Autodesk Fusion 360 part; units mm, degrees
sketch "Sketch5" plane through (0, 0, 0) normal (0, 0, 1) x (1, 0, 0)
  line L0 (9.3481, 1.8494) -> (4.1024, 1.8494)
  line L1 (9.3481, -1.8494) -> (4.1024, -1.8494)
  arc A0 (9.2519, -1.8494) -> (9.2519, 1.8494) centre (9.3, 0) ccw
  arc A1 (4.1024, 1.8494) -> (4.1024, -1.8494) centre (0, 0) ccw
  dimension "d23" = 9
  dimension "d24" = 3.7
  dimension "d25" = 9.3
sketch "Sketch6" plane through (0, 0, 0) normal (0, 0, 1) x (1, 0, 0)
  circle A0 centre (0, 0) radius 1.7
  dimension "d26" = 3.4
extrude "Extrude6" add sketch "Sketch5" against normal blind 2.7
hole "Hole2" at (0, 0, 0) direction (0, 0, -1) diameter 3.4 depth 2.7 tip angle 118
sketch "Sketch7" plane through (0, 0, 0) normal (0, 0, 1) x (1, 0, 0)
  circle A0 centre (9.3, 0) radius 1.55
  dimension "d32" = 3.1
  dimension "d33" = 9.3
extrude "Extrude7" add sketch "Sketch7" along normal blind 10.4
sketch "Sketch1" plane through (0, 0, 0) normal (0, 0, 1) x (1, 0, 0)
  circle A0 centre (0, 0) radius 10.7065
  dimension "d1" = 21.413
extrude "Extrude1" [suppressed]
sketch "Sketch2" plane through (0, 0, 0) normal (0, 0, 1) x (1, 0, 0)
  circle A0 centre (0, 0) radius 1.5
  dimension "d4" = 3
sketch "Sketch3" plane through (0, 0, 0) normal (0, 0, 1) x (1, 0, 0)
  circle A0 centre (0, 0) radius 1.5
  circle A1 centre (7.5, 0) radius 1.5
  dimension "d7" = 3
  dimension "d9" = 3
  dimension "d10" = 7.5
sketch "Sketch4" plane through (0, 0, 0) normal (0, 0, 1) x (1, 0, 0)
  circle A0 centre (0, 0) radius 1.5
  dimension "d8" = 3
extrude "Extrude3" [suppressed]
hole "Hole1" [suppressed]
extrude "Extrude4" [suppressed]
extrude "Extrude5" [suppressed]
split "Split1" [suppressed]
Work out the finished part from the listing and answer in its coordinate system (mm). A direction names the side the tool comes from. Coordinates: 2 decimals unless noted, no trailing zeros. Loops run counter-clockwise (first coordinate to the right, second up) from the corner with the lowest first, then second, coordinate; pieces in that order, holes last. Notation, with made-up numbers: (8, 86.5) - (42, 86.5) arc R20 ccw to (42, 97.5) - close; hole circle Ø1 at (-35.75, 26). An arc over 180 degrees is marked (long way). Use a Markdown table: item, result.
Item 1: For faces 1 (the cylindrical face through (10.778, -0.466, 5.127)), 2 (the flat face through (1.5, 1.1, -2.7)), 3 (the flat face through (7, -1.849, -1)), determine the directions among +Z, -Z, +X, -X, +Y, -Y from which every point of the face is accessible in a straight line to the end or side of a thin tool.
Evaluation:
| item | result |
|---|---|
| face 1 | +Z |
| face 2 | -Z, +X, -X, +Y, -Y |
| face 3 | +Z, -Z, +X, -Y |
Item 2: Find section A-A, the plane x = 0. Determine the outline of the cut face in (y, z), and give its area (3 significant figures).
Evaluation:
| item | result |
|---|---|
| outline | (-4.5, -2.7) - (-1.7, -2.7) - (-1.7, 0) - (-4.5, 0) - close; (1.7, -2.7) - (4.5, -2.7) - (4.5, 0) - (1.7, 0) - close |
| area | 15.1 mm2 |
Item 3: Find section D-D, the plane y = -1. Determine the outline of the cut face in (x, z).
Evaluation:
| item | result |
|---|---|
| outline | (-4.39, -2.7) - (-1.37, -2.7) - (-1.37, 0) - (-4.39, 0) - close; (1.37, -2.7) - (10.86, -2.7) - (10.86, 0) - (10.48, 0) - (10.48, 10.4) - (8.12, 10.4) - (8.12, 0) - (1.37, 0) - close |
Item 4: Given pin 1 Ø4 at (y, z) = (2, 2.5) entering from -X; pin 2 Ø1.5 at (y, z) = (-1.5, 3) entering from +X; pin 3 Ø1.4 at (x, z) = (6.5, -0.5) entering from +Y, each flat-ended and moving along its own axis, determine where each tip first touches the part or whether it passes through.
Evaluation:
| item | result |
|---|---|
| pin 1 | stops at x = 7.75 |
| pin 2 | stops at x = 10.66 |
| pin 3 | stops at y = 1.85 |
Item 5: Find section C-C, the plane z = 1. Determine the outline of the cut face in (x, y), and give its area (3 significant figures).
Evaluation:
| item | result |
|---|---|
| outline | circle Ø3.1 at (9.3, 0) |
| area | 7.55 mm2 |
Item 6: The mould has two halves that part along Y. Classify faces 4 (the cylindrical face through (1.66, 0.37, -1.37)), 5 (the flat face through (7, 1.849, -1)), 6 (the flat face through (1.5, 1.1, 0)): +Y half, -Y half, draft (parallel to the pull), parting line (faces both ways), or undercut.
Evaluation:
| item | result |
|---|---|
| face 4 | undercut |
| face 5 | +Y half |
| face 6 | draft |
Item 7: Consider probe 1 along X at (y, z) = (0, -1.95); probe 2 along Y at (x, z) = (0, -1.1); probe 3 along Z at (x, y) = (3.5, 1.5). Determine where each line is inside the solid, lowest interval first. Write a range as from..to.
Evaluation:
| item | result |
|---|---|
| probe 1 | x = -4.5..-1.7, 1.7..11.15 |
| probe 2 | y = -4.5..-1.7, 1.7..4.5 |
| probe 3 | z = -2.7..0 |
Item 8: Find section B-B, the plane y = 0. Determine the outline of the cut face in (x, z), and give its area (3 significant figures).
Evaluation:
| item | result |
|---|---|
| outline | (-4.5, -2.7) - (-1.7, -2.7) - (-1.7, 0) - (-4.5, 0) - close; (1.7, -2.7) - (11.15, -2.7) - (11.15, 0) - (10.85, 0) - (10.85, 10.4) - (7.75, 10.4) - (7.75, 0) - (1.7, 0) - close |
| area | 65.3 mm2 |
